The listing builds one solid part. Answer for the finished solid, in the listing's coordinates (mm). A direction names the side the tool comes from. Coordinates: 2 decimals unless noted, no trailing zeros. Order: outer loops, then holes, each group sorted by start corner. A loop starts at its lowest first (then second) coordinate and runs counter-clockwise, first axis right, second up. Notation, with made-up numbers: (61, 27.5) -> (91, 27.5) arc R8 ccw to (91, 35.5) -> close; hole circle Ø6 at (26, 84.25). An arc over 180 degrees is marked (long way). Return JSON: item names as keys, results as strings.
```python
from build123d import *

# Parameters (mm, degrees)
F0_W       = 30
F0_H       = 110
F0_R       = 2.5
F1_DEPTH   = 5
F2_R       = 10
F3_R       = 6
F3_R_2     = 5
F4_DEPTH   = 1
F5_W       = 10
F5_H       = 5
F6_DEPTH   = 20
F7_W       = 10
F7_H       = 10
F8_DEPTH   = 55
F9_W       = 109.809534
F9_H       = 10
F10_DEPTH  = 80
F10_FACE_W = 90
F10_FACE_H = 10
F11_DEPTH  = 50
F13_DEPTH  = 10
F15_DEPTH  = 10


with BuildPart() as f1:
    # F0 (on Top) → F1 (new body)
    with BuildSketch(Plane.XY):
        with Locations((-53.017432, -53.040362)):
            Rectangle(F0_W, F0_H)
        with Locations((-53.017432, -95.540362)):
            Circle(F0_R, mode=Mode.SUBTRACT)
        with Locations((-53.017432, -10.540362)):
            Circle(F0_R, mode=Mode.SUBTRACT)
    extrude(amount=F1_DEPTH)

    # F2
    f2_edges = [f1.edges().sort_by_distance(p)[0] for p in [
        (-68.017432, -108.040362, 2.5),
        (-68.017432, 1.959638, 2.5),
    ]]
    fillet(f2_edges, radius=F2_R)

    # F3 (on face) → F4 (join)
    with BuildSketch(Plane.XY.offset(5)):
        with Locations((-53.017432, -10.540362)):
            Circle(F3_R)
        with Locations((-53.017432, -10.540362)):
            Circle(F3_R_2, mode=Mode.SUBTRACT)
        with Locations((-53.017432, -95.540362)):
            Circle(F3_R)
        with Locations((-53.017432, -95.540362)):
            Circle(F3_R_2, mode=Mode.SUBTRACT)
    extrude(amount=F4_DEPTH)

    # F5 (on face) → F6 (join)
    with BuildSketch(Plane.YZ.offset(-38.017432)):
        with Locations((-103.040362, 2.5)):
            Rectangle(F5_W, F5_H)
        with Locations((-3.040362, 2.5)):
            Rectangle(F5_W, F5_H)
    extrude(amount=F6_DEPTH)

    # F7 (on face) → F8 (join)
    with BuildSketch(Plane(origin=(0, 0, 0), x_dir=(1, 0, 0), z_dir=(0, 0, -1))):
        with Locations((-23.017432, 3.040362)):
            Rectangle(F7_W, F7_H)
        with Locations((-23.017432, 103.040362)):
            Rectangle(F7_W, F7_H)
    extrude(amount=F8_DEPTH)

    # F9 (on face) → F10 (join)
    with BuildSketch(Plane.YZ.offset(-18.017432)):
        with Locations((-52.945129, -50)):
            Rectangle(F9_W, F9_H)
    extrude(amount=F10_DEPTH)

    # F10_face (on face) → F11 (cut)
    with BuildSketch(Plane(origin=(-18.017432, -53.040362, -50), x_dir=(0, 1, 0), z_dir=(-1, 0, 0))):
        Rectangle(F10_FACE_W, F10_FACE_H)
    extrude(amount=-F11_DEPTH, mode=Mode.SUBTRACT)

    # F12 (on face) → F13 (join)
    with BuildSketch(Plane(origin=(0, 1.959638, 0), x_dir=(-1, 0, 0), z_dir=(0, 1, 0))):
        Polygon((18.017432, -5), (18.017432, 5), (-61.982568, -45), (-51.982568, -45), align=None)
    extrude(amount=-F13_DEPTH)

    # F14 (on face) → F15 (join)
    with BuildSketch(Plane(origin=(0, -98.040362, 0), x_dir=(-1, 0, 0), z_dir=(0, 1, 0))):
        Polygon((18.017432, -5), (18.017432, 5), (-61.925042, -45), (-51.925042, -45), align=None)
    extrude(amount=-F15_DEPTH)


solid = f1.part
```
Item 1: The part is cut by section C-C on x = 22. Determine the outline of the cut face in (y, z).
Answer list:
{"outline": "(-108.04, -27.89) -> (-98.04, -27.89) -> (-98.04, -20.03) -> (-108.04, -20.03) -> close; (-107.85, -55) -> (-98.04, -55) -> (-98.04, -45) -> (-107.85, -45) -> close; (-8.04, -55) -> (1.96, -55) -> (1.96, -45) -> (-8.04, -45) -> close; (-8.04, -27.87) -> (1.96, -27.87) -> (1.96, -20.01) -> (-8.04, -20.01) -> close"}
Item 2: Find the intervals of material crossed by probe 1 along Y at (x, z) = (18.5, -51); probe 2 along Y at (x, z) = (-26, -9); probe 3 along Z at (x, y) = (-48, -7), in increasing order.
Answer list:
{"probe 1": "-107.85 to -98.04, -8.04 to 1.96", "probe 2": "-108.04 to -98.04, -8.04 to 1.96", "probe 3": "0 to 5"}
Item 3: The part is cut by section B-B on z = -8. Determine the outline of the cut face in (x, y), plus the area to 3 significant figures.
Answer list:
{"outline": "(-28.02, -108.04) -> (-18.02, -108.04) -> (-18.02, -98.04) -> (-28.02, -98.04) -> close; (-28.02, -8.04) -> (-18.02, -8.04) -> (-18.02, 1.96) -> (-28.02, 1.96) -> close; (-12.77, -108.04) -> (2.77, -108.04) -> (2.77, -98.04) -> (-12.77, -98.04) -> close; (-12.77, -8.04) -> (2.78, -8.04) -> (2.78, 1.96) -> (-12.77, 1.96) -> close", "area": "511 mm2"}
Item 4: Determine the mould class of faces 1 (the flat face through (5, -8.04, -16)), 2 (the cylindrical face through (-65.2, -105, 2.5)), 3 (the flat face through (17.44, -102.97, -25.28)), 4 (the cylindrical face through (-53.34, -93.06, 2.46)) for opening direction X: pulls with the +X half, pulls with the -X half, needs draft (parallel to the pull), parting line crosses it, or undercut.
Answer list:
{"face 1": "needs draft", "face 2": "pulls with the -X half", "face 3": "undercut", "face 4": "undercut"}
Item 5: The part is cut by section D-D on z = -47.5. Determine the outline of the cut face in (x, y).
Answer list:
{"outline": "(-28.02, -108.04) -> (-18.02, -108.04) -> (-18.02, -107.85) -> (61.98, -107.85) -> (61.98, 1.96) -> (-28.02, 1.96) -> (-28.02, -8.04) -> (31.98, -8.04) -> (31.98, -98.04) -> (-28.02, -98.04) -> close"}
Item 6: Flat-ended cylindrical pins translate along their axes: pin 1 (6 mm diameter, centred on x = -9, z = -47, fed in from -Y); pin 2 (16 mm diameter, centred on x = -53.02, y = -95.54, fed in from -Z); pin 3 (3 mm diameter, centred on y = -4.5, z = -16, fed in from +X). Find the tip coordinate at first contact, or state that the pin passes through.
Answer list:
{"pin 1": "y = -107.85", "pin 2": "z = 0", "pin 3": "x = 17.98"}
Item 7: Which of the six approach directions +Z, -Z, +X, -X, +Y, -Y give full straight-line access (tool end or side, diameter ignored) to faces 5 (the flat face through (-53, -54, 0)), 6 (the flat face through (39, -54, -45)), 7 (the flat face through (21, -107.85, -50))?
Answer list:
{"face 5": "-Z, -X, +Y, -Y", "face 6": "none", "face 7": "-Z, +X, -Y"}
Item 8: The part is cut by section A-A on y = -46.5. Determine the outline of the cut face in (x, z).
Answer list:
{"outline": "(-68.02, 0) -> (-38.02, 0) -> (-38.02, 5) -> (-68.02, 5) -> close; (31.98, -55) -> (61.98, -55) -> (61.98, -45) -> (31.98, -45) -> close"}
